Job drawing, mm, ordinate dimensions from the low corner. One solid piece. A direction names the side the tool comes from. Round coordinates to 2 decimals unless told otherwise and drop trailing zeros. Loops run counter-clockwise (first coordinate to the right, second up) from the corner with the lowest first, then second, coordinate; pieces in that order, holes last.
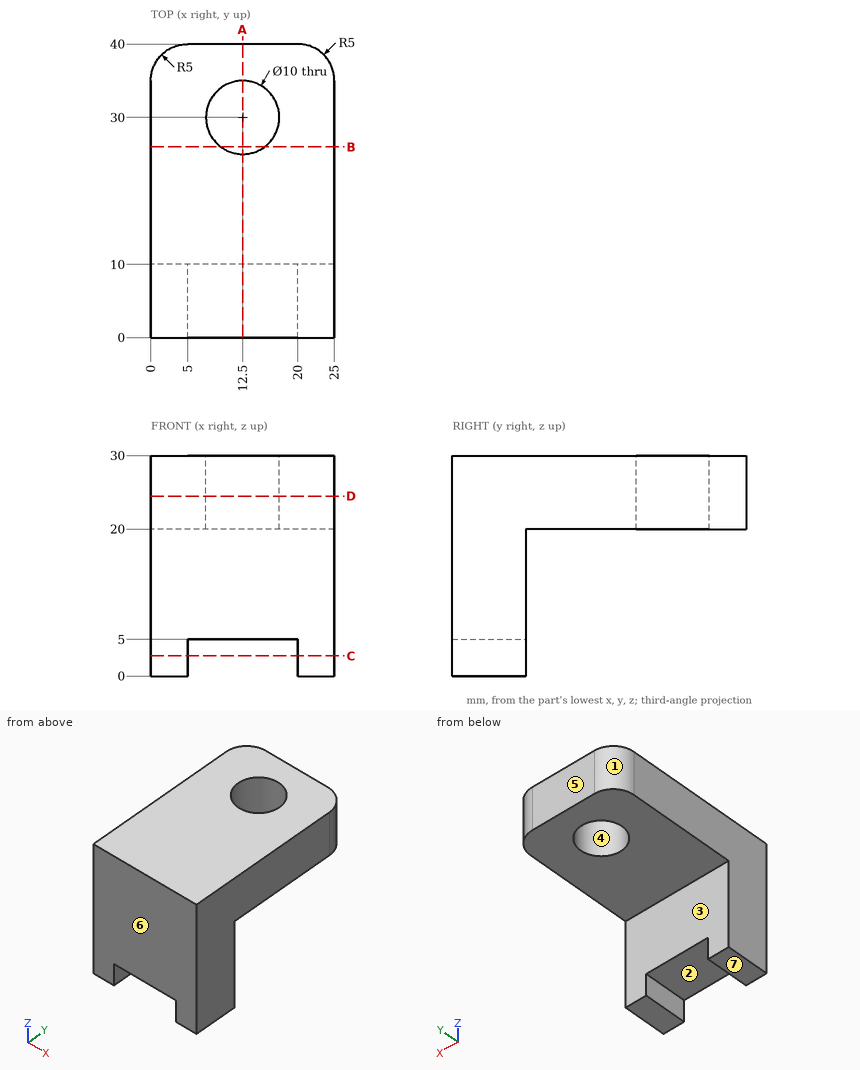
Item 1: Probe line 1 (Y direction, x = 12.5, z = 27.25); line 2 (Z direction, x = 4, y = 37.5); line 3 (Y direction, x = 23.25, z = 6.75). List the from-to ranges inside material, lowest first.
Answers follow:
line 1: y = 0 to 25, 35 to 40
line 2: z = 20 to 30
line 3: y = 0 to 10
Item 2: Cut at D-D, the plane z = 24.5. Give the cut face in (x, y).
Answers follow:
outline: (0, 0) - (25, 0) - (25, 35) arc R5 ccw to (20, 40) - (5, 40) arc R5 ccw to (0, 35) - close; hole circle Ø10 at (12.5, 30)
Item 3: Cut at A-A, the plane x = 12.5. Give the cut face in (y, z).
Answers follow:
outline: (0, 5) - (10, 5) - (10, 20) - (25, 20) - (25, 30) - (0, 30) - close; (35, 20) - (40, 20) - (40, 30) - (35, 30) - close
Item 4: Flat gauge pins, fed straight in: P1, Ø1.5, axis at x = 6.5, y = 5.5, coming from the -Z side; P2, Ø10, axis at x = 16.5, z = 8, coming from the +Y side; P3, Ø5, axis at x = 16.5, y = 19, coming from the -Z side. Where does each tip first touch, or does it go through?
Answers follow:
P1: stops at z = 5
P2: stops at y = 10
P3: stops at z = 20
Item 5: Cut at B-B, the plane y = 26. Give the cut face in (x, z), plus the area to 3 significant figures.
Answers follow:
outline: (0, 20) - (9.5, 20) - (9.5, 30) - (0, 30) - close; (15.5, 20) - (25, 20) - (25, 30) - (15.5, 30) - close
area: 190 mm2
Item 6: Cut at C-C, the plane z = 2.75. Give the cut face in (x, y), plus the area to 3 significant figures.
Answers follow:
outline: (0, 0) - (5, 0) - (5, 10) - (0, 10) - close; (20, 0) - (25, 0) - (25, 10) - (20, 10) - close
area: 100 mm2
Item 7: Two-plate mould, pull along Y, no slides. Class the marked faces 4, 5, 6 and 7: released by +Y, released by -Y, zero draft, split by the parting line, or undercut.
Answers follow:
face 4: undercut
face 5: released by +Y
face 6: released by -Y
face 7: zero draft
Item 8: 3-axis set-ups, long thin cutter, end or side, ignore diameter. For the marked faces 1, 2 and 3: which of +Z, -Z, +X, -X, +Y, -Y reach the whole face in a straight line?
Answers follow:
face 1: +Z, -Z, -X, +Y
face 2: -Z, +Y, -Y
face 3: -Z, +X, -X, +Y
